Design review of the part built by this model. Coordinates are the model's own, in mm. A direction names the side the tool comes from. Round coordinates to 2 decimals unless told otherwise and drop trailing zeros. Loops run counter-clockwise (first coordinate to the right, second up) from the corner with the lowest first, then second, coordinate; pieces in that order, holes last. Notation, with made-up numbers: (-20, 69) - (4, 69) arc R25 cw to (4, 99) - close; hole circle Ø11 at (8.5, 86.25). An arc over 180 degrees is marked (long way). Answer as CSV lines item,"result". Start each with the question number.
(1) For faces 1 (the flat face through (36, 49, -1028.7)), 2 (the flat face through (35.322, 35, 14)), list the 3-axis set-ups (+Z, -Z, +X, -X, +Y, -Y) from which the entire face can be reached by the end or side of a thin tool; tool diameter is ignored.
(2) Consider section A-A (z = 756). Give the boundary of the cut face in (x, y), and give its area (3 significant figures).
(3) Consider section B-B (x = 10). Give the boundary of the cut face in (y, z).
(4) For P1, Ø1.5, axis at y = 11, z = -181.5, coming from the -X side; P2, Ø4, axis at x = 28.5, z = -662.5, coming from the -Y side; P3, Ø4, axis at x = 19.05, z = -933.45, coming from the -Y side; P4, Ø7.5, axis at x = 19.05, z = -504.825, coming from the +Y side, all flat-tipped, find the tip position at first contact; note any pin that passes through.
(5) Consider section C-C (y = 53). Give the boundary of the cut face in (x, z).
(6) Wall thickness on L1, parallel to X at y = 72.9, z = 666.75 (3 decimals); L2, parallel to Y at x = 13, z = 443.5; L3, parallel to X at y = 68, z = -17: over which ranges is each line inside the solid? List them lowest first.
from build123d import *

# Parameters (mm, degrees)
F0_W     = 38.1
F0_H     = 74.6125
F1_DEPTH = 1028.7
F2_T     = -2.778125
F3_R     = 3.175
F4_DEPTH = 74.6135


with BuildPart() as f1:
    # F0 (on Top) → F1 (new body, symmetric)
    with BuildSketch(Plane.XY):
        with Locations((19.05, 37.30625)):
            Rectangle(F0_W, F0_H)
    extrude(amount=F1_DEPTH, both=True)

    # F2
    f2_openings = [f1.faces().sort_by_distance(p)[0] for p in [
        (19.05, 37.30625, 1028.7),
        (19.05, 0, 0),
        (19.05, 37.30625, -1028.7),
        (0, 37.30625, 0),
    ]]
    offset(amount=F2_T, openings=f2_openings)

    # F3 (on face) → F4 (cut, through all)
    with BuildSketch(Plane(origin=(0, 74.6125, 0), x_dir=(-1, 0, 0), z_dir=(0, 1, 0))):
        with Locations((-19.05, 561.975)):
            Circle(F3_R)
        with Locations((-19.05, 511.175)):
            Circle(F3_R)
        with Locations((-19.05, 133.35)):
            Circle(F3_R)
        with Locations((-19.05, -22.225)):
            Circle(F3_R)
        with Locations((-19.05, 28.575)):
            Circle(F3_R)
        with Locations((-19.05, -400.05)):
            Circle(F3_R)
        with Locations((-19.05, -555.625)):
            Circle(F3_R)
        with Locations((-19.05, -504.825)):
            Circle(F3_R)
        with Locations((-19.05, -933.45)):
            Circle(F3_R)
        with Locations((-19.05, 666.75)):
            Circle(F3_R)
        with Locations((-19.05, 1009.65)):
            Circle(F3_R)
    extrude(amount=-F4_DEPTH, mode=Mode.SUBTRACT)


solid = f1.part
Determined:
1,face 1,"-Z, +X, -X, +Y, -Y"
1,face 2,"+Z, -Z, -X, -Y"
2,outline,"(0, 71.83) - (35.32, 71.83) - (35.32, 0) - (38.1, 0) - (38.1, 74.61) - (0, 74.61) - close"
2,area,"305 mm^2"
3,outline,"(71.83, -1028.7) - (74.61, -1028.7) - (74.61, 1028.7) - (71.83, 1028.7) - close"
4,P1,"stops at x = 35.32"
4,P2,"stops at y = 71.83"
4,P3,"passes through"
4,P4,"stops at y = 74.61"
5,outline,"(35.32, -1028.7) - (38.1, -1028.7) - (38.1, 1028.7) - (35.32, 1028.7) - close"
6,L1,"x = 0 to 15.875, 22.225 to 38.1"
6,L2,"y = 71.83 to 74.61"
6,L3,"x = 35.32 to 38.1"
